Could you check a few things on this model? Use its own coordinates, in mm. A direction names the side the tool comes from. Round coordinates to 2 decimals unless told otherwise and drop trailing zeros. Loops run counter-clockwise (first coordinate to the right, second up) from the corner with the lowest first, then second, coordinate; pieces in that order, holes last.
from build123d import *

# Parameters (mm, degrees)
PAD_DEPTH = 10


with BuildPart() as part:
    # Sketch → Pad (new body)
    with BuildSketch(Plane.XY):
        with BuildLine():
            ThreePointArc((-8.268256, 22.633972), (-12.815763, 18.086465), (-8.268256, 13.538958))
            Line((9.182689, 13.538958), (-8.268256, 13.538958))
            ThreePointArc((9.182689, 8.443945), (11.730196, 10.991452), (9.182689, 13.538958))
            Line((9.182689, 8.443945), (3.547507, 8.443945))
            ThreePointArc((3.547507, 8.443945), (0.331934, 7.112011), (-1, 3.896438))
            Line((-1, -6.103562), (-1, 3.896438))
            Line((1, -6.103562), (-1, -6.103562))
            Line((1, 3.896438), (1, -6.103562))
            ThreePointArc((3.547507, 6.443945), (1.746147, 5.697797), (1, 3.896438))
            Line((3.547507, 6.443945), (9.182689, 6.443945))
            ThreePointArc((9.182689, 6.443945), (13.730196, 10.991452), (9.182689, 15.538958))
            Line((-8.268256, 15.538958), (9.182689, 15.538958))
            ThreePointArc((-8.268256, 20.633972), (-10.815763, 18.086465), (-8.268256, 15.538958))
            Line((-8.268256, 20.633972), (9.182689, 20.633972))
            ThreePointArc((9.182689, 20.633972), (13.730196, 25.181478), (9.182689, 29.728985))
            Line((-8.268256, 29.728985), (9.182689, 29.728985))
            ThreePointArc((-8.268256, 34.823999), (-10.815763, 32.276492), (-8.268256, 29.728985))
            Line((-8.268256, 34.823999), (8.568406, 34.823999))
            ThreePointArc((8.568406, 34.823999), (13.115912, 39.371505), (8.568406, 43.919012))
            Line((8.568406, 43.919012), (3.547507, 43.919012))
            ThreePointArc((1, 46.466519), (1.746147, 44.66516), (3.547507, 43.919012))
            Line((1, 56.466519), (1, 46.466519))
            Line((-1, 56.466519), (1, 56.466519))
            Line((-1, 46.466519), (-1, 56.466519))
            ThreePointArc((-1, 46.466519), (0.331934, 43.250946), (3.547507, 41.919012))
            Line((8.568406, 41.919012), (3.547507, 41.919012))
            ThreePointArc((8.568406, 36.823999), (11.115912, 39.371505), (8.568406, 41.919012))
            Line((-8.268256, 36.823999), (8.568406, 36.823999))
            ThreePointArc((-8.268256, 36.823999), (-12.815763, 32.276492), (-8.268256, 27.728985))
            Line((9.182689, 27.728985), (-8.268256, 27.728985))
            ThreePointArc((9.182689, 22.633972), (11.730196, 25.181478), (9.182689, 27.728985))
            Line((-8.268256, 22.633972), (9.182689, 22.633972))
        make_face()
    extrude(amount=PAD_DEPTH)


solid = part.part
Item 1: For faces 5 (the flat face through (6, 43.919, 5)), 6 (the flat face through (1, 27.729, 5)), 7 (the flat face through (0, 20.634, 5)), 8 (the flat face through (2, 21, 10)), which set-ups out of +Z, -Z, +X, -X, +Y, -Y let a thin tool reach every point of the face, with its end or its side?
Results list:
face 5: +Z, -Z, +X, +Y
face 6: +Z, -Z, -X
face 7: +Z, -Z, +X
face 8: +Z, +X, -X, +Y, -Y
Item 2: If we section it at B-B, the plane y = -1.5: Please give me the cut outline in (x, z).
Results list:
outline: (-1, 0) - (1, 0) - (1, 10) - (-1, 10) - close
Item 3: If I drill on line 1 along Y through (x, z) = (5.75, 2.5); line 2 along Y through (x, z) = (-7.5, 6.75); line 3 along Y through (x, z) = (3, 4.75), over which ranges is the centre line in solid material (lowest first)?
Results list:
line 1: y = 6.44 to 8.44, 13.54 to 15.54, 20.63 to 22.63, 27.73 to 29.73, 34.82 to 36.82, 41.92 to 43.92
line 2: y = 13.54 to 15.54, 20.63 to 22.63, 27.73 to 29.73, 34.82 to 36.82
line 3: y = 6.38 to 8.41, 13.54 to 15.54, 20.63 to 22.63, 27.73 to 29.73, 34.82 to 36.82, 41.95 to 43.98
Item 4: If we section it at C-C, the plane y = 43: Please give me the cut outline in (x, z), then the cut area to 3 significant figures.
Results list:
outline: (0.6, 0) - (11.31, 0) - (11.31, 10) - (0.6, 10) - close
area: 107 mm2
Item 5: Will these pins go through, and if not, where does the flat tip stop? pin 1 (5 mm diameter, centred on y = 0.5, z = 5.5, fed in from +X); pin 2 (1.5 mm diameter, centred on x = 5.5, z = 4.5, fed in from +Y); pin 3 (1.5 mm diameter, centred on x = -3.5, z = 7, fed in from -Y); pin 4 (1.5 mm diameter, centred on x = 11, y = 31.5, fed in from -Z).
Results list:
pin 1: stops at x = 1
pin 2: stops at y = 43.92
pin 3: stops at y = 13.54
pin 4: passes through
Item 6: We'd pull the mould along Y, two halves only. Please class faces 1 (the cylindrical face through (1.726, 44.685, 4.93)), 2 (the cylindrical face through (-12.815, 18.186, 4.93)), 3 (the flat face through (2, 21, 0)), 4 (the cylindrical face through (-10.815, 18.142, 4.93)): released by +Y, released by -Y, zero draft, split by the parting line, or undercut.
Results list:
face 1: released by +Y
face 2: undercut
face 3: zero draft
face 4: undercut
